from build123d import *

# Parameters (mm, degrees)
SKETCH_1_R          = 17.25
EXTRUDE_1_DEPTH     = 13.7
SKETCH_2_R          = 1.25
CUT_EXTRUDE_1_DEPTH = 3
CUT_EXTRUDE_START   = 3
SKETCH_3_R          = 1.25
CUT_EXTRUDE_2_DEPTH = 3
SKETCH_4_R          = 6.25
SKETCH_4_R_2        = 4.25
CUT_EXTRUDE_3_DEPTH = 2
SKETCH_5_R          = 3.25
CUT_EXTRUDE_4_DEPTH = 0.7
FILLET_1_R          = 0.3
SKETCH_6_R          = 3
CUT_EXTRUDE_6_DEPTH = 11


with BuildPart() as part:
    # 草图1 → 凸台-拉伸1 (new body)
    with BuildSketch(Plane.XY):
        with Locations(Location((0, 0, 0), (0, 0, 180))):
            Circle(SKETCH_1_R)
    extrude(amount=EXTRUDE_1_DEPTH)

    # 草图2 → 切除-拉伸1 (cut)
    with BuildSketch(Plane.XY.offset(13.7)):
        with Locations((0, 7.75)):
            Circle(SKETCH_2_R)
        with Locations((7.75, 0)):
            Circle(SKETCH_2_R)
        with Locations((0, -7.75)):
            Circle(SKETCH_2_R)
        with Locations((-7.75, 0)):
            Circle(SKETCH_2_R)
    extrude(amount=-CUT_EXTRUDE_1_DEPTH, mode=Mode.SUBTRACT)

    # 草图3 → 切除-拉伸2 (cut)
    with BuildSketch(Plane.XY.offset(CUT_EXTRUDE_START)):
        with Locations((0, 7.75)):
            Circle(SKETCH_3_R)
        with Locations((7.75, 0)):
            Circle(SKETCH_3_R)
        with Locations((0, -7.75)):
            Circle(SKETCH_3_R)
        with Locations((-7.75, 0)):
            Circle(SKETCH_3_R)
    extrude(amount=-CUT_EXTRUDE_2_DEPTH, mode=Mode.SUBTRACT)

    # 草图4 → 切除-拉伸3 (cut)
    with BuildSketch(Plane.XY):
        Circle(SKETCH_4_R)
        Circle(SKETCH_4_R_2, mode=Mode.SUBTRACT)
    extrude(amount=CUT_EXTRUDE_3_DEPTH, mode=Mode.SUBTRACT)

    # 草图5 → 切除-拉伸4 (cut)
    with BuildSketch(Plane.XY):
        Circle(SKETCH_5_R)
    extrude(amount=CUT_EXTRUDE_4_DEPTH, mode=Mode.SUBTRACT)

    # 圆角1
    fillet_1_edges = [part.edges().sort_by_distance(p)[0] for p in [
        (-4.25, 0, 0),
        (-3.25, 0, 0),
    ]]
    fillet(fillet_1_edges, radius=FILLET_1_R)

    # 草图6 → 切除-拉伸6 (cut)
    with BuildSketch(Plane.XY.offset(13.7)):
        Circle(SKETCH_6_R)
    extrude(amount=-CUT_EXTRUDE_6_DEPTH, mode=Mode.SUBTRACT)


solid = part.part
Work out the finished part from the listing and answer in its coordinate system (mm). A direction names the side the tool comes from. Round coordinates to 2 decimals unless told otherwise and drop trailing zeros. Write each loop counter-clockwise with the first axis right and the second up, starting at its lowest first coordinate (ties: lowest second). Pieces come first, ordered by that corner, then holes. Notation, with made-up numbers: (44, 71) - (96, 71) arc R13 cw to (96, 93) - close; hole circle Ø7 at (62.25, 25). An arc over 180 degrees is marked (long way). Answer in a Markdown table with one row per item. Add a question column.
1. For faces 4 (the flat face through (-8, 0, 3)), 5 (the cylindrical face through (0, -9, 12)), determine the directions among +Z, -Z, +X, -X, +Y, -Y from which every point of the face is accessible in a straight line to the end or side of a thin tool.
2. A cutting plane is placed at C-C, the plane y = 5.5. Determine the outline of the cut face in (x, z).
3. A cutting plane is placed at B-B, the plane z = 9. Determine the outline of the cut face in (x, y).
4. Given pin 1 (0.8 mm diameter, centred on x = -8.5, y = 0, fed in from +Z); pin 2 (1.5 mm diameter, centred on x = -7.75, y = 0, fed in from -Z); pin 3 (2 mm diameter, centred on y = 10, z = 4, fed in from +X), each flat-ended and moving along its own axis, determine where each tip first touches the part or whether it passes through.
5. A cutting plane is placed at A-A, the plane z = 1.25. Determine the outline of the cut face in (x, y), and give its area (3 significant figures).
6. The mould has two halves that part along X. Classify faces 1 (the cylindrical face through (17.233, -0.758, 6.754)), 2 (the flat face through (-4, 7, 0)), 3 (the cylindrical face through (-9, 0, 2)): +X half, -X half, draft (parallel to the pull), parting line (faces both ways), or undercut.
7. Find the intervals of material crossed by line 1 along Y through (x, z) = (0, 11.75); line 2 along Y through (x, z) = (0, 1.4); line 3 along X through (y, z) = (-1.5, 7.5), in increasing order. Write a range as from..to.
Worked out:
| question | item | result |
|---|---|---|
| 1 | face 4 | -Z |
| 1 | face 5 | +Z |
| 2 | outline | (-16.35, 0) - (-2.97, 0) - (-2.97, 2) - (2.97, 2) - (2.97, 0) - (16.35, 0) - (16.35, 13.7) - (-16.35, 13.7) - close |
| 3 | outline | circle Ø34.5 at (0, 0); hole circle Ø6 at (0, 0) |
| 4 | pin 1 | z = 10.7 |
| 4 | pin 2 | z = 3 |
| 4 | pin 3 | x = 14.72 |
| 5 | outline | circle Ø34.5 at (0, 0); circle Ø8.5 at (0, 0); hole circle Ø2.5 at (-7.75, 0); hole circle Ø12.5 at (0, 0); hole circle Ø2.5 at (0, -7.75); hole circle Ø2.5 at (0, 7.75); hole circle Ø2.5 at (7.75, 0) |
| 5 | area | 849 mm^2 |
| 6 | face 1 | parting line |
| 6 | face 2 | draft |
| 6 | face 3 | undercut |
| 7 | line 1 | -17.25..-9, -6.5..-3, 3..6.5, 9..17.25 |
| 7 | line 2 | -17.25..-9, -6.5..-6.25, -4.25..4.25, 6.25..6.5, 9..17.25 |
| 7 | line 3 | -17.18..-2.6, 2.6..17.18 |
